Input: dimensioned drawing with shaded views. Units: mm. Origin: part minimum x, y, z. A direction names the side the tool comes from. Round coordinates to 2 decimals unless told otherwise and drop trailing zeros. Loops run counter-clockwise (first coordinate to the right, second up) from the corner with the lowest first, then second, coordinate; pieces in that order, holes last.
Item 1: Access query for the marked faces 1 and 2. Directions: +Z, -Z, +X, -X, +Y, -Y. A direction counts if a zero-diameter tool reaches every point of the face in a straight line with its end or side. Return the directions, or none.
Item 2: Section query C-C on z = 11.43. Return loops of the section in (x, y) (1 decimal).
Item 3: First-contact query: P1, Ø1.5, axis at y = 10, z = 3.5, coming from the +X side; P2, Ø5.5, axis at x = 10.5, y = 7.5, coming from the +Z side. Flat tips, straight axial feed; report the tip coordinate or a pass-through.
Item 4: Ray query, L1, parallel to X at y = 11, z = 13.75; L2, parallel to Y at x = 8.5, z = 0.5. Return the intervals inside material, ascending.
Item 5: Section query D-D on y = 17.5. Return loops of the section in (x, z).
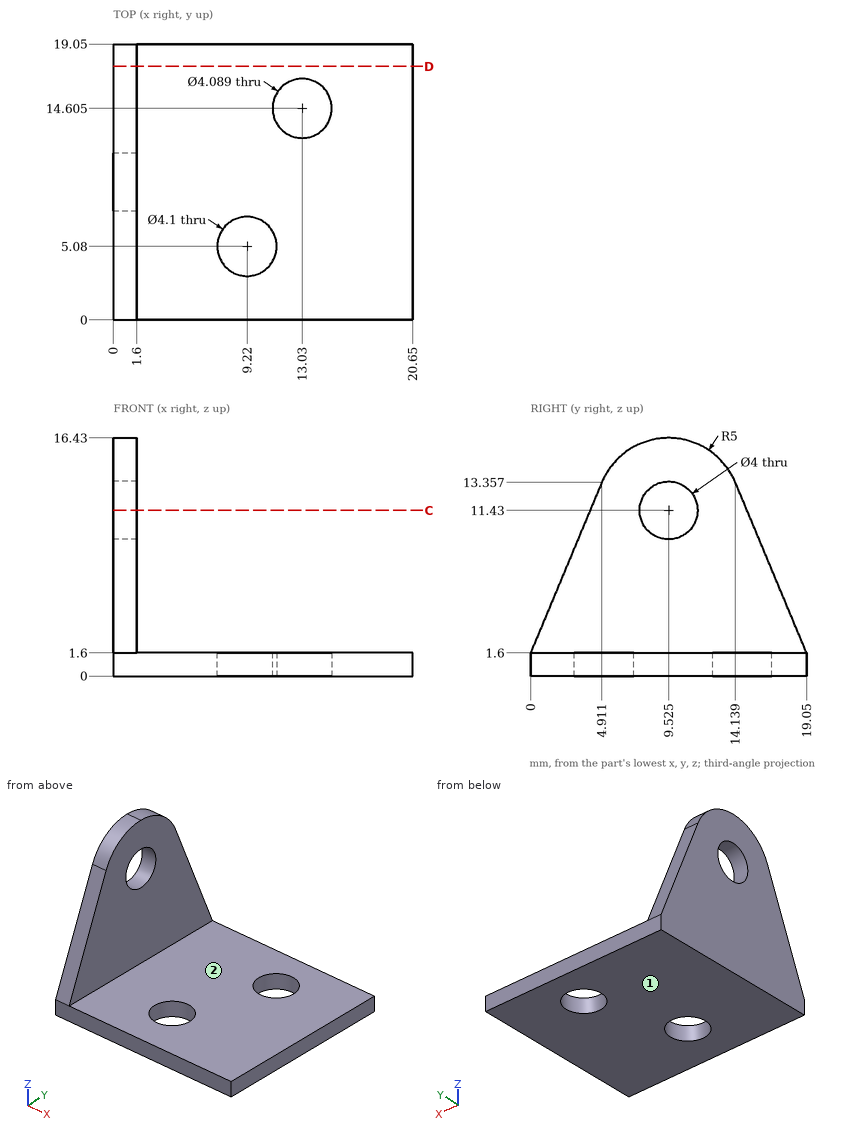
Data:
1. face 1: -Z, +X, -X, +Y, -Y
1. face 2: +Z, +X, +Y, -Y
2. outline: (0, 4.1) - (1.6, 4.1) - (1.6, 7.5) - (0, 7.5) - close; (0, 11.5) - (1.6, 11.5) - (1.6, 14.9) - (0, 14.9) - close
3. P1: stops at x = 1.6
3. P2: stops at z = 1.6
4. L1: x = 0 to 1.6
4. L2: y = 0 to 3.16, 7 to 19.05
5. outline: (0, 0) - (20.65, 0) - (20.65, 1.6) - (1.6, 1.6) - (1.6, 5.31) - (0, 5.31) - close
